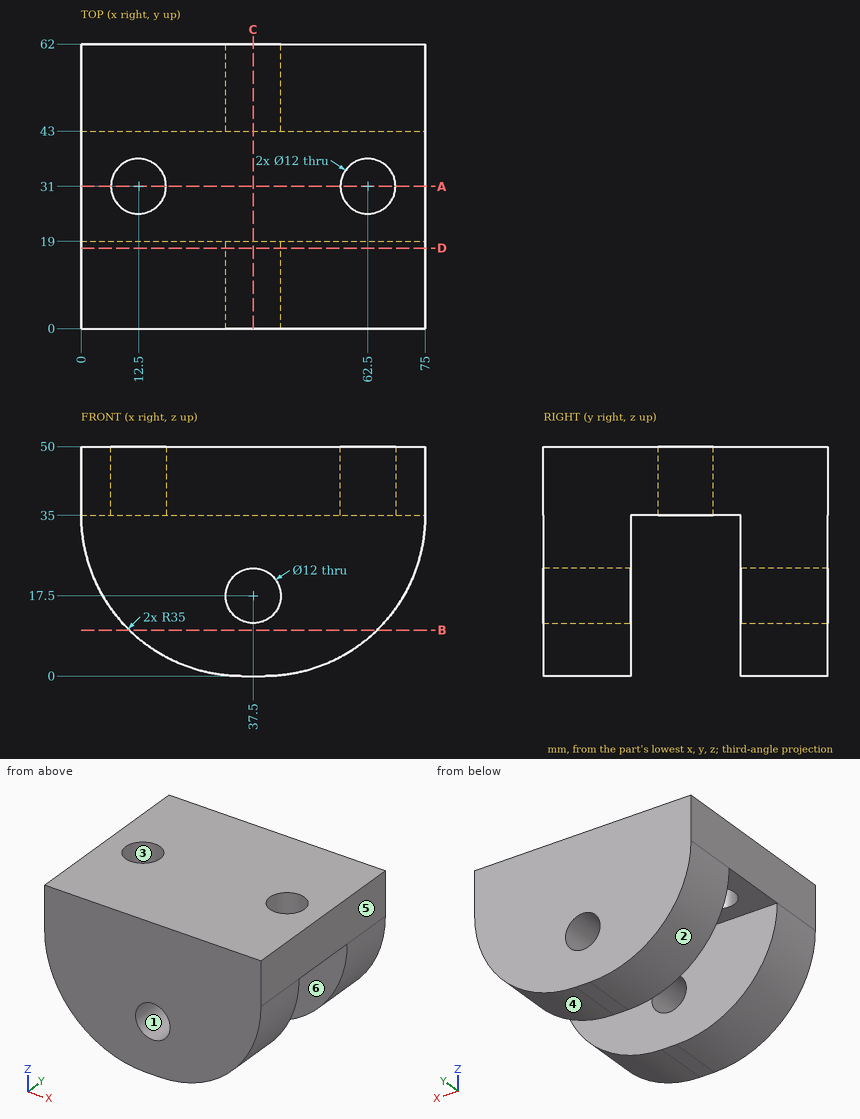
Geometry: see drawing. Coordinates: mm, zero at the bounding-box minimum. A direction names the side the tool comes from. Give positions to 0.01 mm unless a question says otherwise; leave off trailing zeros. Order: outer loops, then holes, each group sorted by start corner. A loop starts at its lowest first (then second) coordinate and runs counter-clockwise, first axis right, second up.
Q1. Section A-A on y = 31. Output: boundary loops of the cut face in (x, z), and give its area (3 significant figures).
Checked values:
outline: (0, 35) - (6.5, 35) - (6.5, 50) - (0, 50) - close; (18.5, 35) - (56.5, 35) - (56.5, 50) - (18.5, 50) - close; (68.5, 35) - (75, 35) - (75, 50) - (68.5, 50) - close
area: 765 mm2
Q2. Set-up query: the marked faces 5 and 6. Return all of +Z, -Z, +X, -X, +Y, -Y with unobstructed straight access to the full face (end or side cutting, diameter ignored); none if empty.
Checked values:
face 5: +Z, -Z, +X, +Y, -Y
face 6: -Z, +X, -X
Q3. Ray query, probe 1 along Y at (x, z) = (25, 25); probe 2 along Y at (x, z) = (62, 39); probe 3 along X at (y, z) = (10.25, 17.5). Return the intervals inside material, ascending.
Checked values:
probe 1: y = 0 to 19, 43 to 62
probe 2: y = 0 to 25.02, 36.98 to 62
probe 3: x = 4.69 to 31.5, 43.5 to 70.31
Q4. Section B-B on z = 10. Output: boundary loops of the cut face in (x, y), and give its area (3 significant figures).
Checked values:
outline: (10.51, 0) - (64.49, 0) - (64.49, 19) - (10.51, 19) - close; (10.51, 43) - (64.49, 43) - (64.49, 62) - (10.51, 62) - close
area: 2,050 mm2
Q5. Contact query for flat-ended pins moving along their axis: pin 1 Ø1.5 at (y, z) = (51, 21.5) entering from +X; pin 2 Ø6 at (x, y) = (28.5, 29) entering from -Z; pin 3 Ø12 at (x, y) = (26.5, 50) entering from -Z. Output: stop coordinate, or through.
Checked values:
pin 1: stops at x = 72.6
pin 2: stops at z = 35
pin 3: stops at z = 0.09
Q6. Section C-C on x = 37.5. Output: boundary loops of the cut face in (y, z), and give its area (3 significant figures).
Checked values:
outline: (0, 0) - (19, 0) - (19, 11.5) - (0, 11.5) - close; (0, 23.5) - (19, 23.5) - (19, 35) - (43, 35) - (43, 23.5) - (62, 23.5) - (62, 50) - (0, 50) - close; (43, 0) - (62, 0) - (62, 11.5) - (43, 11.5) - close
area: 1,800 mm2
Q7. Section D-D on y = 17.5. Output: boundary loops of the cut face in (x, z).
Checked values:
outline: (0, 35) arc R35 ccw to (35, 0) - (40, 0) arc R35 ccw to (75, 35) - (75, 50) - (0, 50) - close; hole circle Ø12 at (37.5, 17.5)
Q8. Draft query along X for the marked faces 1, 2, 3 and 4. Return one class per face: +X half, -X half, draft (parallel to the pull), parting line (faces both ways), or undercut.
Checked values:
face 1: undercut
face 2: -X half
face 3: undercut
face 4: +X half
